The model under review builds one solid part; all positions refer to its coordinate system, in mm. Coordinates: 2 decimals unless noted, no trailing zeros. Loops run counter-clockwise (first coordinate to the right, second up) from the corner with the lowest first, then second, coordinate; pieces in that order, holes last. Notation, with made-up numbers: (63.25, -26) - (91.25, -26) arc R30 ccw to (91.25, -2) - close; hole circle Ø4 at (-17, -22). An arc over 180 degrees is marked (long way). One line per item, written item: value. Start each with the question number.
1. Mouldability with a two-part tool opening along X and no side actions: class faces 1 (the face through (28.19, -110.17, 1.57)), 2 (the face through (148.009, -110.373, 1.565)), 3 (the face through (159.254, -84.426, 1.565)) as +X half, -X half, draft (parallel to the pull), parting line (faces both ways), or undercut.
2. To check wall thickness, follow line 1 (X direction, y = -117.5, z = 2.5); line 2 (Y direction, x = 78.5, z = 0.6); line 3 (Y direction, x = 105, z = 0.7). State the ranges of each line that lie inside material, in increasing order.
3. We need section B-B, the plane z = 1.2. Count the separate pieces of the cut face and the enclosed holes in it, then the cut area to 3 significant figures.
4. Insertion check: P1, Ø6, axis at x = 28.68, y = -122.37, coming from the +Z side (3 decimals); P2, Ø1, axis at x = 92, z = 2, coming from the -Y side; P3, Ø1, axis at x = 126, z = 1, coming from the -Y side; P4, Ø1.5, axis at y = -31, z = 2.5, coming from the +X side. Each pin has a flat end and moves straight along its axis. Give the tip position at first contact, or say it passes through.
5. We need section C-C, the plane x = 10. Give the boundary of the cut face in (y, z) (3 decimals).
6. We need section A-A, the plane x = 64.5. Give the boundary of the cut face in (y, z) (3 decimals).
Autodesk Inventor part; units mm, degrees
ref_plane "YZ Plane" through (0, 0, 0) normal (1, 0, 0) x (0, 1, 0)
ref_plane "XZ Plane" through (0, 0, 0) normal (0, 1, 0) x (-1, 0, 0)
ref_plane "XY Plane" through (0, 0, 0) normal (0, 0, 1) x (1, 0, 0)
sketch "Sketch1" plane through (0, 0, 0) normal (0, 0, 1) x (1, 0, 0)
  arc A0 (16.121808, -110.692366) -> (67.383886, -131.656361) centre (43.321682, -117.338179) ccw
  line L0 (67.383886, -131.656361) -> (108.159478, -131.656361)
  arc A1 (108.159478, -131.656361) -> (139.594615, -90.326332) centre (132.221682, -117.338179) ccw
  arc A2 (132.227805, -80.679244) -> (139.594615, -90.326332) centre (142.227805, -80.679244) ccw
  line L1 (132.227805, -80.679244) -> (132.227805, -71.827)
  arc A3 (132.227805, -71.827) -> (90.658044, -1.487819) centre (51.933317, -71.827) ccw
  arc A4 (90.658044, -1.487819) -> (84.870639, 0) centre (84.870639, -12) ccw
  line L2 (84.870639, 0) -> (0, 0)
  line L3 (0, 0) -> (0, -88.644145)
  arc A5 (0, -88.644145) -> (8.203784, -98.481503) centre (10, -88.644145) ccw
  arc A6 (16.121808, -110.692366) -> (8.203784, -98.481503) centre (6.407567, -108.318861) ccw
  circle A7 centre (121.188208, -82.443861) radius 3.3
  arc A8 (145.794404, -114.286904) -> (148.095336, -110.420107) centre (146.970651, -112.368846) ccw
  circle A9 centre (97.470651, -122.368861) radius 2.25
  circle A10 centre (97.470651, -112.368852) radius 2.25
  circle A11 centre (78.175839, -122.368861) radius 2.25
  arc A12 (145.794404, -124.286918) -> (148.095336, -120.420122) centre (146.970651, -122.368861) ccw
  circle A13 centre (22.617078, -8.511936) radius 2.8
  circle A14 centre (22.617078, -40.511936) radius 2.8
  circle A15 centre (28.675839, -122.368861) radius 2.25
  circle A16 centre (28.675837, -112.368861) radius 2.25
  circle A17 centre (78.175837, -112.368855) radius 2.25
  circle A18 centre (10, -88.644145) radius 3.3
  line L4 (73.060526, -128.291526) -> (33.526976, -128.291526)
  arc A19 (32.526976, -127.291526) -> (33.526976, -128.291526) centre (33.526976, -127.291526) ccw
  line L5 (32.526976, -127.291526) -> (32.526973, -107.491526)
  arc A20 (33.526973, -106.491526) -> (32.526973, -107.491526) centre (33.526973, -107.491526) ccw
  line L6 (33.526973, -106.491526) -> (73.060526, -106.491526)
  arc A21 (74.060526, -107.491526) -> (73.060526, -106.491526) centre (73.060526, -107.491526) ccw
  line L7 (74.060526, -107.491526) -> (74.060526, -127.291526)
  arc A22 (73.060526, -128.291526) -> (74.060526, -127.291526) centre (73.060526, -127.291526) ccw
  line L8 (142.119512, -128.291526) -> (102.585962, -128.291526)
  arc A23 (101.585962, -127.291526) -> (102.585962, -128.291526) centre (102.585962, -127.291526) ccw
  line L9 (101.585962, -127.291526) -> (101.585962, -107.491526)
  arc A24 (102.585962, -106.491526) -> (101.585962, -107.491526) centre (102.585962, -107.491526) ccw
  line L10 (102.585962, -106.491526) -> (142.119515, -106.491526)
  arc A25 (143.119515, -107.491526) -> (142.119515, -106.491526) centre (142.119515, -107.491526) ccw
  line L11 (143.119515, -107.491526) -> (143.119512, -127.291526)
  arc A26 (142.119512, -128.291526) -> (143.119512, -127.291526) centre (142.119512, -127.291526) ccw
  circle A27 centre (146.970651, -112.368846) radius 2.25
  circle A28 centre (146.970651, -122.368861) radius 2.25
  line L12 (28.675837, -112.368861) -> (146.970651, -112.368846) construction
  line L13 (28.675839, -122.368861) -> (146.970651, -122.368861) construction
  circle A29 centre (43.373245, -117.368861) radius 6
  line L14 (67.43545, -131.687043) -> (108.211041, -131.687043)
  arc A30 (108.211041, -131.687043) -> (160.273251, -117.36885) centre (132.273245, -117.36885) ccw
  line L15 (160.273251, -117.36885) -> (160.273251, -88.823719)
  arc A31 (160.273251, -88.823719) -> (156.504028, -81.00212) centre (150.273251, -88.823719) ccw
  line L16 (156.504028, -81.00212) -> (134.936633, -63.821281)
  arc A32 (131.322196, -57.752321) -> (134.936633, -63.821281) centre (141.167411, -55.999682) ccw
  arc A33 (131.322196, -57.752321) -> (90.995274, -1.485865) centre (52.270547, -71.825046) ccw
  arc A34 (90.995274, -1.485865) -> (85.207869, 0.001954) centre (85.207869, -11.998046) ccw
  line L17 (85.207869, 0.001954) -> (0.051563, 0.001954)
  line L18 (0.051563, 0.001954) -> (0.051563, -88.674827)
  arc A35 (0.051563, -88.674827) -> (8.255347, -98.512185) centre (10.051563, -88.674827) ccw
  arc A36 (16.173371, -110.723048) -> (8.255347, -98.512185) centre (6.45913, -108.349543) ccw
  arc A37 (16.173371, -110.723048) -> (67.43545, -131.687043) centre (43.373245, -117.368861) ccw
  circle A38 centre (22.617078, -40.511936) radius 2.8
  circle A39 centre (22.617078, -8.511936) radius 2.8
  circle A40 centre (155.051563, -88.644145) radius 3.3
  circle A41 centre (10.051563, -88.644145) radius 3.3
  circle A42 centre (132.273245, -117.36885) radius 6
  circle A43 centre (78.175837, -21.998046) radius 3.25
  circle A44 centre (78.175837, -21.998046) radius 6
  point P0 (58.854578, -117.368861)
  point P1 (148.095336, -110.420107)
  point P2 (117.931008, -141.41673)
  point P3 (0.051563, 0)
  dimension "d2" = 49.5
  dimension "d3" = 49.5
  dimension "d4" = 49.5
  dimension "d5" = 49.5
  dimension "d6" = 10
  dimension "d7" = 12
  dimension "d8" = 22
sketch "Sketch1 outline for Extrusion1" plane through (0, 0, 0) normal (0, 0, 1) x (1, 0, 0)
  line L0 (85.207869, 0.001954) -> (0, 0)
  line L1 (0, 0) -> (0, -88.644145)
  arc A0 (0, -88.644145) -> (8.203784, -98.481503) centre (10, -88.644145) ccw
  arc A1 (8.203784, -98.481503) -> (16.121808, -110.692366) centre (6.407567, -108.318861) cw
  arc A2 (16.121808, -110.692366) -> (67.383886, -131.656361) centre (43.321682, -117.338179) ccw
  line L2 (67.383886, -131.656361) -> (108.159478, -131.656361)
  arc A3 (108.159478, -131.656361) -> (117.931008, -141.41673) centre (132.221682, -117.338179) ccw
  arc A4 (117.931008, -141.41673) -> (160.273251, -117.36885) centre (132.273245, -117.36885) ccw
  line L3 (160.273251, -117.36885) -> (160.273251, -88.823719)
  arc A5 (160.273251, -88.823719) -> (156.504028, -81.00212) centre (150.273251, -88.823719) ccw
  line L4 (156.504028, -81.00212) -> (134.936633, -63.821281)
  arc A6 (134.936633, -63.821281) -> (131.322196, -57.752321) centre (141.167411, -55.999682) cw
  arc A7 (131.322196, -57.752321) -> (90.995274, -1.485865) centre (52.270547, -71.825046) ccw
  arc A8 (90.995274, -1.485865) -> (85.207869, 0.001954) centre (85.207869, -11.998046) ccw
  circle A9 centre (155.051563, -88.644145) radius 3.3
  circle A10 centre (78.175837, -21.998046) radius 6
  circle A11 centre (22.617078, -8.511936) radius 2.8
  circle A12 centre (22.617078, -40.511936) radius 2.8
  circle A13 centre (146.970651, -112.368846) radius 2.25
  circle A14 centre (28.675839, -122.368861) radius 2.25
  circle A15 centre (28.675837, -112.368861) radius 2.25
  line L5 (74.060526, -107.491526) -> (74.060526, -127.291526)
  arc A16 (74.060526, -127.291526) -> (73.060526, -128.291526) centre (73.060526, -127.291526) cw
  line L6 (73.060526, -128.291526) -> (33.526976, -128.291526)
  arc A17 (33.526976, -128.291526) -> (32.526976, -127.291526) centre (33.526976, -127.291526) cw
  line L7 (32.526976, -127.291526) -> (32.526973, -107.491526)
  arc A18 (32.526973, -107.491526) -> (33.526973, -106.491526) centre (33.526973, -107.491526) cw
  line L8 (33.526973, -106.491526) -> (73.060526, -106.491526)
  arc A19 (73.060526, -106.491526) -> (74.060526, -107.491526) centre (73.060526, -107.491526) cw
  circle A20 centre (10, -88.644145) radius 3.3
  circle A21 centre (78.175839, -122.368861) radius 2.25
  circle A22 centre (97.470651, -122.368861) radius 2.25
  circle A23 centre (78.175837, -112.368855) radius 2.25
  circle A24 centre (97.470651, -112.368852) radius 2.25
  line L9 (102.585962, -106.491526) -> (142.119515, -106.491526)
  arc A25 (142.119515, -106.491526) -> (143.119515, -107.491526) centre (142.119515, -107.491526) cw
  line L10 (143.119515, -107.491526) -> (143.119512, -127.291526)
  arc A26 (143.119512, -127.291526) -> (142.119512, -128.291526) centre (142.119512, -127.291526) cw
  line L11 (142.119512, -128.291526) -> (102.585962, -128.291526)
  arc A27 (102.585962, -128.291526) -> (101.585962, -127.291526) centre (102.585962, -127.291526) cw
  line L12 (101.585962, -127.291526) -> (101.585962, -107.491526)
  arc A28 (101.585962, -107.491526) -> (102.585962, -106.491526) centre (102.585962, -107.491526) cw
  circle A29 centre (146.970651, -122.368861) radius 2.25
extrude "Extrusion1" add sketch "Sketch1 outline for Extrusion1" along normal blind 3.175
properties part number "Intake Sides V4_servo" material "Polycarbonate, Clear"
Findings below:
1. face 1: undercut
1. face 2: undercut
1. face 3: +X half
2. line 1: 15.32 to 32.53, 74.06 to 101.59, 143.12 to 160.27
2. line 2: -131.66 to -124.6, -120.14 to -114.6, -110.14 to -27.99, -16.01 to 0
2. line 3: -131.66 to -128.29, -106.49 to -11.27
3. separate pieces: 1
3. enclosed holes: 15
3. area: 16,400 mm2
4. P1: z = 3.175
4. P2: y = -131.66
4. P3: y = -144.77
4. P4: x = 121.85
5. outline: (-98.986, 0) - (-91.944, 0) - (-91.944, 3.175) - (-98.986, 3.175) - close; (-85.344, 0) - (0, 0) - (0, 3.175) - (-85.344, 3.175) - close
6. outline: (-135.654, 0) - (-128.292, 0) - (-128.292, 3.175) - (-135.654, 3.175) - close; (-106.492, 0) - (0.001, 0) - (0.001, 3.175) - (-106.492, 3.175) - close
